from build123d import *

# Parameters (mm, degrees)
SKETCH1_R               = 12.9921
BOSS_EXTRUDE1_DEPTH     = 25.4
CUT_EXTRUDE1_DEPTH      = 71.405666164
CUT_EXTRUDE1_DEPTH_BACK = 71.405666164
SKETCH3_R               = 3.81
SKETCH6_R               = 8.255
CUT_EXTRUDE2_DEPTH      = 2.032


with BuildPart() as part:
    # Sketch1 → Boss-Extrude1 (new body)
    with BuildSketch(Plane(origin=(0, 0, 0), x_dir=(1, 0, 0), z_dir=(0, 1, 0))):
        with Locations(Location((0, 0, 0), (0, 0, 270))):
            Circle(SKETCH1_R)
    extrude(amount=BOSS_EXTRUDE1_DEPTH)

    # Sketch2 → Revolve1 (revolve)
    with BuildSketch(Plane(origin=(0, 0, 0), x_dir=(0, 0, -1), z_dir=(1, 0, 0))):
        with BuildLine():
            Line((-16.764, 25.4), (-16.764, 49.53))
            ThreePointArc((-16.764, 49.53), (-11.85393808, 61.38393808), (0, 66.294))
            Line((0, 66.294), (0, 25.4))
            Line((0, 25.4), (-16.764, 25.4))
        make_face()
    revolve(axis=Axis((0, 25.4, 0), (0, 1, 0)))

    # Sketch3 → Cut-Extrude1 (cut, two sides: drawn at the far end of the back side and taken through both)
    with BuildSketch(Plane(origin=(0, 0, 0), x_dir=(0, 0, -1), z_dir=(1, 0, 0)).offset(-CUT_EXTRUDE1_DEPTH_BACK)):
        with Locations((0, 49.53)):
            Circle(SKETCH3_R)
    extrude(amount=CUT_EXTRUDE1_DEPTH + CUT_EXTRUDE1_DEPTH_BACK, mode=Mode.SUBTRACT)

    # Sketch4 → Cut-Revolve1 (revolve, cut)
    with BuildSketch(Plane.XY, mode=Mode.PRIVATE) as cut_revolve1_sk:
        with BuildLine():
            Line((-7.62, 32.995439638), (-7.62, 49.53))
            Line((-7.62, 49.53), (7.62, 49.53))
            Line((7.62, 49.53), (7.62, 32.995439638))
            ThreePointArc((7.62, 32.995439638), (0, 31.32406453), (-7.62, 32.995439638))
        make_face()
    revolve(cut_revolve1_sk.sketch.rotate(Axis((-7.62, 49.53, 0), (1, 0, 0)), 90), axis=Axis((-7.62, 49.53, 0), (1, 0, 0)), mode=Mode.SUBTRACT)

    # Sketch6 → Cut-Extrude2 (cut)
    with BuildSketch(Plane(origin=(16.764, 0, 0), x_dir=(0, 0, -1), z_dir=(1, 0, 0))):
        with Locations((0, 49.53)):
            Circle(SKETCH6_R)
    cut_extrude2 = extrude(amount=-CUT_EXTRUDE2_DEPTH, mode=Mode.SUBTRACT)

    # Mirror1: Cut-Extrude2 across plane
    add(cut_extrude2.mirror(Plane(origin=(0, 0, 0), x_dir=(0, 0, 1), z_dir=(1, 0, 0))), mode=Mode.SUBTRACT)


solid = part.part
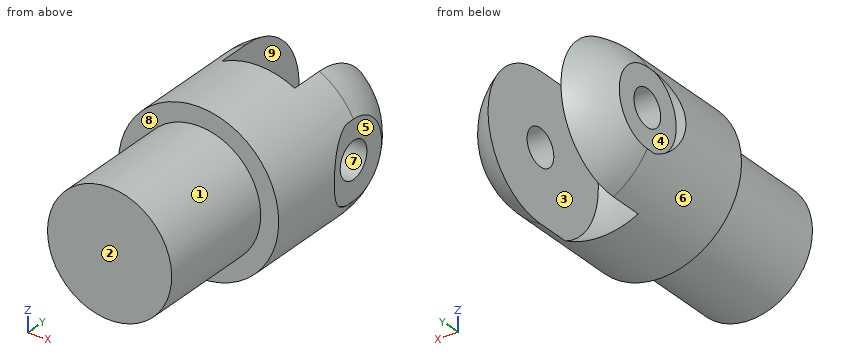
Here's how the part is built. I have some questions about the finished solid (model axes, mm). Face numbers are marked on the shaded views. A direction names the side the tool comes from. Coordinates: 2 decimals unless noted, no trailing zeros. Order: outer loops, then holes, each group sorted by start corner. A loop starts at its lowest first (then second) coordinate and runs counter-clockwise, first axis right, second up. Notation, with made-up numbers: (62.5, 54.5) -> (119.5, 54.5) arc R5 cw to (119.5, 58.5) -> close; hole circle Ø11 at (11, -3.5). An arc over 180 degrees is marked (long way). Answer in a Markdown table with one row per item.
(1) I want a section at B-B on x = 12. List the corners of the cut face in (y, z) for me, then the cut area to 3 significant figures.
Answer key:
| item | result |
|---|---|
| outline | (0, -4.98) -> (25.4, -4.98) -> (25.4, -11.71) -> (49.53, -11.71) arc R11.71 ccw to (49.53, 11.71) -> (25.4, 11.71) -> (25.4, 4.98) -> (0, 4.98) -> close; hole circle Ø7.62 at (49.53, 0) |
| area | 988 mm^2 |
(2) I want a section at D-D on z = -5.5. List the corners of the cut face in (x, y) for me.
Answer key:
| item | result |
|---|---|
| outline | (-15.84, 25.4) -> (-11.77, 25.4) -> (-11.77, 0) -> (11.77, 0) -> (11.77, 25.4) -> (15.84, 25.4) -> (15.84, 43.37) -> (14.73, 43.37) -> (14.73, 55.34) arc R15.84 ccw to (7.62, 63.41) -> (7.62, 33.94) arc R17.36 cw to (-7.62, 33.94) -> (-7.62, 63.41) arc R15.84 ccw to (-14.73, 55.34) -> (-14.73, 43.37) -> (-15.84, 43.37) -> close |
(3) On a 3-axis mill with a long thin cutter (end or side, diameter ignored), from which of +Z, -Z, +X, -X, +Y, -Y can I reach the whole of each face in a straight line? I mean the marked faces 1, 2, 3, 4 and 5. Say none if no direction works.
Answer key:
| item | result |
|---|---|
| face 1 | -Y |
| face 2 | +Z, -Z, +X, -X, -Y |
| face 3 | +Y |
| face 4 | -X, +Y |
| face 5 | +X, +Y |
(4) I want a section at A-A on z = 0. List the corners of the cut face in (x, y) for me (3 decimals).
Answer key:
| item | result |
|---|---|
| outline | (-16.764, 25.4) -> (-12.992, 25.4) -> (-12.992, 0) -> (12.992, 0) -> (12.992, 25.4) -> (16.764, 25.4) -> (16.764, 41.275) -> (14.732, 41.275) -> (14.732, 45.72) -> (7.62, 45.72) -> (7.62, 32.995) arc R18.206 cw to (-7.62, 32.995) -> (-7.62, 45.72) -> (-14.732, 45.72) -> (-14.732, 41.275) -> (-16.764, 41.275) -> close; (-14.732, 53.34) -> (-7.62, 53.34) -> (-7.62, 64.462) arc R16.764 ccw to (-14.732, 57.53) -> close; (7.62, 53.34) -> (14.732, 53.34) -> (14.732, 57.53) arc R16.764 ccw to (7.62, 64.462) -> close |
(5) Thinking about a two-plate mould opening in Z: for the marked faces 6, 7, 8 and 9, which applies, +Z half, -Z half, draft (parallel to the pull), parting line (faces both ways), or undercut?
Answer key:
| item | result |
|---|---|
| face 6 | parting line |
| face 7 | undercut |
| face 8 | draft |
| face 9 | undercut |
(6) Please list where these lines run through material, in increasing order: probe 1 along X at (y, z) = (45.5, -3.5); probe 2 along Z at (x, y) = (11.5, 49.53); probe 3 along X at (y, z) = (39.5, 14).
Answer key:
| item | result |
|---|---|
| probe 1 | -14.73 to -7.62, 7.62 to 14.73 |
| probe 2 | -12.2 to -3.81, 3.81 to 12.2 |
| probe 3 | -9.22 to -5.9, 5.9 to 9.22 |
(7) Will these pins go through, and if not, where does the flat tip stop? pin 1 Ø1 at (y, z) = (27.5, 9.5) entering from +X; pin 2 Ø5 at (x, y) = (4.5, 32) entering from -Z; pin 3 Ø2 at (x, y) = (7.5, 14.5) entering from +Z.
Answer key:
| item | result |
|---|---|
| pin 1 | x = 14.14 |
| pin 2 | z = -16.64 |
| pin 3 | z = 11.25 |
(8) I want a section at C-C on x = 0. List the corners of the cut face in (y, z) for me, then the cut area to 3 significant figures.
Answer key:
| item | result |
|---|---|
| outline | (0, -12.99) -> (25.4, -12.99) -> (25.4, -16.76) -> (42.43, -16.76) arc R18.21 cw to (42.43, 16.76) -> (25.4, 16.76) -> (25.4, 12.99) -> (0, 12.99) -> close |
| area | 962 mm^2 |
